CAD build for the part. Positions are in the model's coordinates, mm. Face numbers are marked on the shaded views. A direction names the side the tool comes from. Round coordinates to 2 decimals unless told otherwise and drop trailing zeros. Order: outer loops, then holes, each group sorted by start corner. A loop starts at its lowest first (then second) coordinate and runs counter-clockwise, first axis right, second up. Notation, with made-up numbers: M 3.25,49.25 L 62.25,49.25 A22 cw 62.25,84.25 Z; hole C 72.5,8 d2. An arc over 180 degrees is marked long. Answer as a JSON object with one key per item and string values.
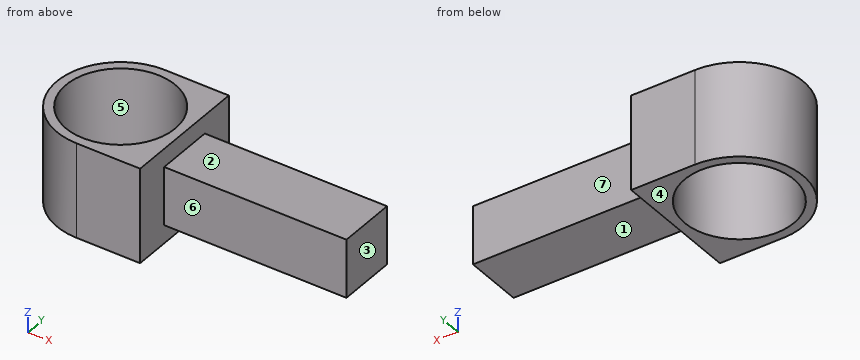
```python
from build123d import *

# Parameters (mm, degrees)
EXTRUDE_1_DEPTH     = 26
SKETCH_2_R          = 15
CUT_EXTRUDE_1_DEPTH = 26
SKETCH_3_W          = 16
SKETCH_3_H          = 16
EXTRUDE_2_DEPTH     = 50


with BuildPart() as part:
    # 草图1 → 凸台-拉伸1 (new body)
    with BuildSketch(Plane.XY):
        with BuildLine():
            Line((0, 17.5), (17.5, 17.5))
            Line((17.5, 17.5), (17.5, -17.5))
            Line((17.5, -17.5), (0, -17.5))
            ThreePointArc((0, -17.5), (-17.5, 0), (0, 17.5))
        make_face()
    extrude(amount=EXTRUDE_1_DEPTH)

    # 草图2 → 切除-拉伸1 (cut)
    with BuildSketch(Plane.XY.offset(26)):
        Circle(SKETCH_2_R)
    extrude(amount=-CUT_EXTRUDE_1_DEPTH, mode=Mode.SUBTRACT)

    # 草图3 → 凸台-拉伸2 (add)
    with BuildSketch(Plane(origin=(17.5, 0, 0), x_dir=(0, 0, -1), z_dir=(1, 0, 0))):
        with Locations((-13, 0)):
            Rectangle(SKETCH_3_W, SKETCH_3_H)
    extrude(amount=EXTRUDE_2_DEPTH)


solid = part.part
```
Item 1: 3-axis set-ups, long thin cutter, end or side, ignore diameter. For the marked faces 1, 2 and 3: which of +Z, -Z, +X, -X, +Y, -Y reach the whole face in a straight line?
Worked answers:
{"face 1": "-Z, +X, +Y, -Y", "face 2": "+Z, +X, +Y, -Y", "face 3": "+Z, -Z, +X, +Y, -Y"}
Item 2: Saw through at A-A on y = 0. List the corners of the cut face in (x, z).
Worked answers:
{"outline": "M -17.5,0 L -15,0 L -15,26 L -17.5,26 Z; M 15,0 L 17.5,0 L 17.5,5 L 67.5,5 L 67.5,21 L 17.5,21 L 17.5,26 L 15,26 Z"}
Item 3: Drop flat-ended pins along their axis: pin 1 Ø8 at (x, y) = (48, -2) entering from -Z; pin 2 Ø12 at (x, z) = (46.5, 20.5) entering from +Y; pin 3 Ø12 at (x, z) = (33.5, 10.5) entering from -Y; pin 4 Ø1 at (x, z) = (41, 3.5) entering from -Y. Give the stop position or say it passes through.
Worked answers:
{"pin 1": "stops at z = 5", "pin 2": "stops at y = 8", "pin 3": "stops at y = -8", "pin 4": "passes through"}
Item 4: Two-plate mould, pull along Y, no slides. Class the marked faces 4, 5, 6 and 7: released by +Y, released by -Y, zero draft, split by the parting line, or undercut.
Worked answers:
{"face 4": "zero draft", "face 5": "undercut", "face 6": "released by -Y", "face 7": "released by +Y"}
Item 5: Wall check: line 1 along Y through (x, z) = (0, 16); line 2 along X through (y, z) = (6.5, 20.5); line 3 along Z through (x, y) = (25.5, -5). Give the ranges that are in metal, low to high. Write a range as [from, to].
Worked answers:
{"line 1": "y = [-17.5, -15], [15, 17.5]", "line 2": "x = [-16.25, -13.52], [13.52, 67.5]", "line 3": "z = [5, 21]"}
Item 6: Saw through at D-D on y = 3.5. List the corners of the cut face in (x, z), and give its area (3 significant figures).
Worked answers:
{"outline": "M -17.15,0 L -14.59,0 L -14.59,26 L -17.15,26 Z; M 14.59,0 L 17.5,0 L 17.5,5 L 67.5,5 L 67.5,21 L 17.5,21 L 17.5,26 L 14.59,26 Z", "area": "942 mm2"}
Item 7: Saw through at C-C on x = -10. List the corners of the cut face in (y, z), and give its area (3 significant figures).
Worked answers:
{"outline": "M -14.36,0 L -11.18,0 L -11.18,26 L -14.36,26 Z; M 11.18,0 L 14.36,0 L 14.36,26 L 11.18,26 Z", "area": "165 mm2"}
Item 8: Saw through at B-B on z = 24.75. List the corners of the cut face in (x, y).
Worked answers:
{"outline": "M 0,-17.5 L 17.5,-17.5 L 17.5,17.5 L 0,17.5 A17.5 ccw Z; hole C 0,0 d30"}
